Input: dimensioned drawing with shaded views. Units: mm. Origin: part minimum x, y, z. A direction names the side the tool comes from. Give positions to 0.01 mm unless a question says otherwise; leave off trailing zeros. Order: outer loops, then holes, each group sorted by start corner. A loop starts at its lowest first (then second) coordinate and runs counter-clockwise, first axis right, second up. Notation, with made-up numbers: (69.5, -18) - (88.5, -18) arc R37 ccw to (88.5, 20) - close; hole circle Ø9 at (50, -24). An arc over 180 degrees is marked (long way). Use a Markdown table: item, result.
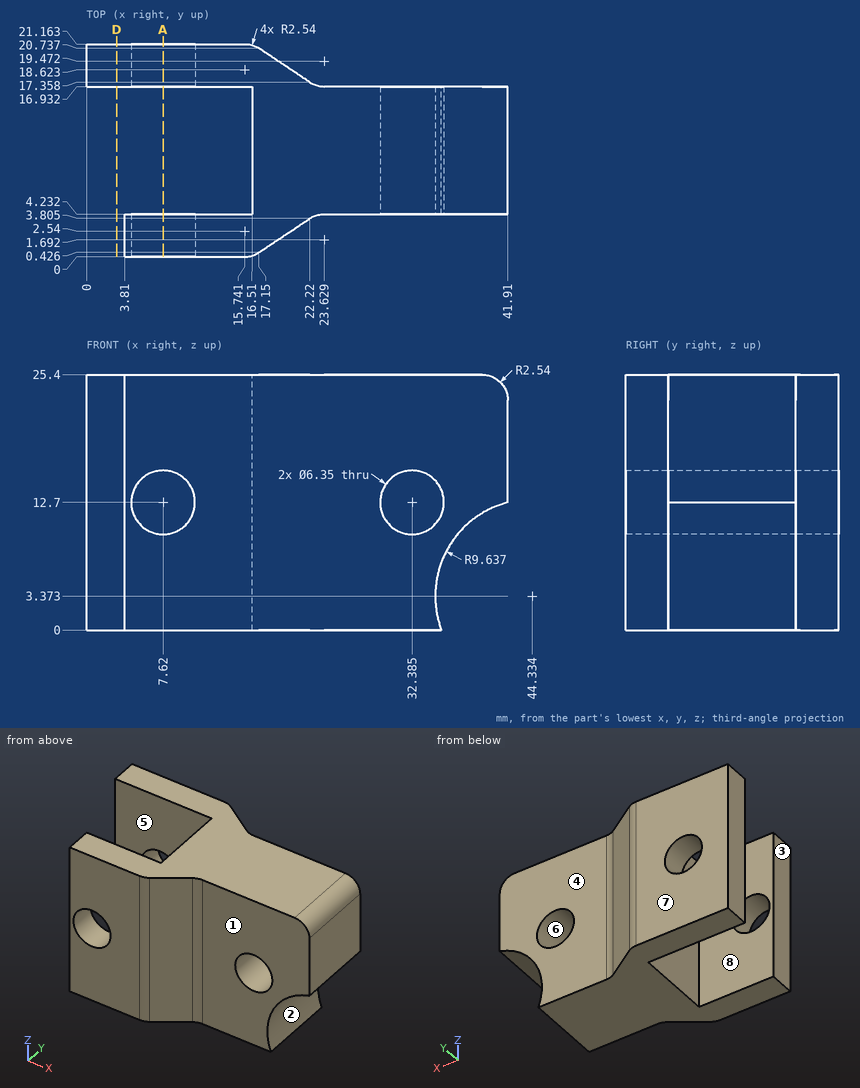
1. Mould query, pull axis Y, two halves, no side actions, for the marked faces 6, 7 and 8. Classes: pulls with the +Y half, pulls with the -Y half, needs draft (parallel to the pull), parting line crosses it, or undercut.
Response:
| item | result |
|---|---|
| face 6 | needs draft |
| face 7 | pulls with the +Y half |
| face 8 | undercut |
2. Pin query (flat end, axial travel): pin 1 (1.3 mm diameter, centred on y = 3, z = 9, fed in from -X); pin 2 (12 mm diameter, centred on x = 5, y = 6.5, fed in from +Z); pin 3 (4 mm diameter, centred on y = 9, z = 9, fed in from -X); pin 4 (1 mm diameter, centred on x = 37, z = 13.5, fed in from -Y). Return the tip coordinate at first contact, or that it passes through.
Response:
| item | result |
|---|---|
| pin 1 | stops at x = 3.81 |
| pin 2 | stops at z = 25.4 |
| pin 3 | stops at x = 16.51 |
| pin 4 | stops at y = 4.23 |
3. Section query D-D (x = 3). Return loops of the section in (y, z).
Response:
| item | result |
|---|---|
| outline | (16.93, 0) - (21.16, 0) - (21.16, 25.4) - (16.93, 25.4) - close |
4. Material intervals for line 1 along Z through (x, y) = (7.62, 3.05) (1 decimal); line 2 along Y through (x, z) = (12, 4.5); line 3 along Y through (x, z) = (3, 16), sorted ascending.
Response:
| item | result |
|---|---|
| line 1 | z = 0 to 9.5, 15.9 to 25.4 |
| line 2 | y = 0 to 4.23, 16.93 to 21.16 |
| line 3 | y = 16.93 to 21.16 |
5. Section query A-A (x = 7.62). Return loops of the section in (y, z) (1 decimal), then the cut area to 3 significant figures.
Response:
| item | result |
|---|---|
| outline | (0, 0) - (4.2, 0) - (4.2, 9.5) - (0, 9.5) - close; (0, 15.9) - (4.2, 15.9) - (4.2, 25.4) - (0, 25.4) - close; (16.9, 0) - (21.2, 0) - (21.2, 9.5) - (16.9, 9.5) - close; (16.9, 15.9) - (21.2, 15.9) - (21.2, 25.4) - (16.9, 25.4) - close |
| area | 161 mm^2 |
6. Set-up query: the marked faces 1, 2, 3, 4 and 5. Return all of +Z, -Z, +X, -X, +Y, -Y with unobstructed straight access to the full face (end or side cutting, diameter ignored); none if empty.
Response:
| item | result |
|---|---|
| face 1 | +Z, -Z, +X, -Y |
| face 2 | +X, +Y, -Y |
| face 3 | +Z, -Z, -X, -Y |
| face 4 | +Z, -Z, +X, +Y |
| face 5 | +Z, -Z, -X |
